Could you check a few things on this model? Use its own coordinates, in mm. Face numbers are marked on the shaded views. A direction names the side the tool comes from. Coordinates: 2 decimals unless noted, no trailing zeros. Loops run counter-clockwise (first coordinate to the right, second up) from the corner with the lowest first, then second, coordinate; pieces in that order, holes last. Notation, with made-up numbers: M 56.5,-16 L 114.5,-16 A8 ccw 114.5,-3 Z; hole C -38.5,23.5 d1. An arc over 180 degrees is marked long. Return JSON: item names as keys, results as strings. Group by question number.
from build123d import *

# Parameters (mm, degrees)
F0_W      = 38.1
F0_H      = 38.1
F1_DEPTH  = 38.1
F6_DEPTH  = 38.1
F8_DEPTH  = 38.1
F9_W      = 25.4
F9_H      = 7.62
F10_DEPTH = 38.1


with BuildPart() as f1:
    # F0 (on Front) → F1 (new body)
    with BuildSketch(Plane.XZ):
        with Locations((19.05, 19.05)):
            Rectangle(F0_W, F0_H)
    extrude(amount=F1_DEPTH)

    # F5 (on offset) → F6 (cut)
    with BuildSketch(Plane.YZ.offset(38.1)):
        Polygon((-11.43, 16.449932), (-6.35, 38.1), (-31.75, 38.1), (-26.67, 16.449932), (-21.59, 28.575), (-16.51, 28.575), align=None)
        Polygon((-6.35, 0), (0, 0), (0, 38.1), align=None)
        Polygon((-19.05, 0), (-12.7, 0), (-19.05, 15.875), (-25.4, 0), align=None)
        Polygon((-31.75, 0), (-38.1, 38.1), (-38.1, 0), align=None)
    extrude(amount=-F6_DEPTH, mode=Mode.SUBTRACT)

    # F7 (on offset) → F8 (cut)
    with BuildSketch(Plane.XZ.offset(38.1)):
        Polygon((11.43, 22.225), (6.35, 0), (31.75, 0), (26.67, 22.225), (21.59, 9.525), (16.51, 9.525), align=None)
        Polygon((25.4, 38.1), (12.7, 38.1), (19.05, 22.225), align=None)
        Polygon((31.75, 38.1), (38.1, 0), (38.1, 38.1), align=None)
        Polygon((0, 38.1), (0, 0), (6.35, 38.1), align=None)
    extrude(amount=-F8_DEPTH, mode=Mode.SUBTRACT)

    # F9 (on offset) → F10 (cut)
    with BuildSketch(Plane.XY.offset(38.1)):
        with Locations((12.7, -26.67)):
            Rectangle(F9_W, F9_H)
        with Locations((25.4, -11.43)):
            Rectangle(F9_W, F9_H)
    extrude(amount=-F10_DEPTH, mode=Mode.SUBTRACT)


solid = f1.part
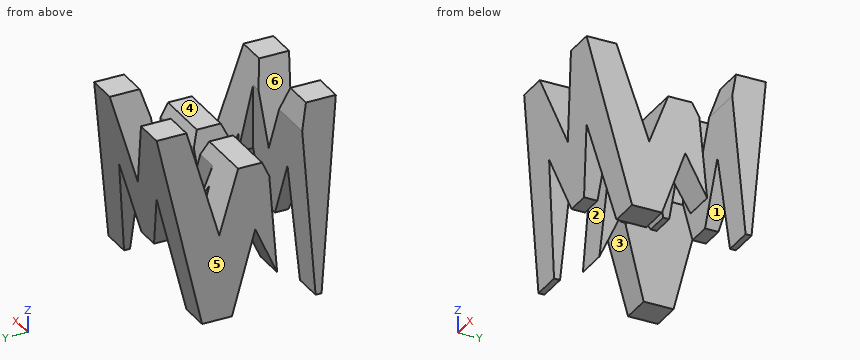
(1) Imagine slicing it at C-C, the plane x = 15.5. Write out the boundary of the cut face in (y, z) (3 decimals).
(2) For the marked faces 1, 2 and 3, which set-ups out of +Z, -Z, +X, -X, +Y, -Y let a thin tool reach every point of the face, with its end or its side?
(3) We'd pull the mould along X, two halves only. Please class the marked faces 4, 5 and 6: +X half, -X half, draft (parallel to the pull), parting line (faces both ways), or undercut.
(4) Will these pins go through, and if not, where does the flat tip stop? P1, Ø5.5, axis at x = 27, y = -18, coming from the +Z side (3 decimals); P2, Ø3.5, axis at y = -29, z = 26, coming from the -X side; P3, Ø1, axis at x = 19.5, y = -15.5, coming from the +Z side.
(5) Imagine slicing it at A-A, the plane z = 35. Write out the boundary of the cut face in (x, y).
(6) If I drill on L1, parallel to Y at x = 5, z = 20; L2, parallel to Y at x = 35, z = 18; L3, parallel to X at y = -32.5, z = 21.5, over which ranges is the centre line in solid material (lowest first)? Write a range as [from, to].
(7) Imagine slicing it at D-D, the plane z = 10.5. Count the separate pieces of the cut face and the enclosed holes in it, then the cut area to 3 significant figures.
Checks:
{
 "1": {"outline": "M -36.933,31.1 L -33.758,12.05 L -30.48,12.05 L -30.48,31.1 Z; M -22.86,12.05 L -20.58,12.05 L -19.05,15.875 L -17.52,12.05 L -15.24,12.05 L -15.24,25.544 L -16.51,28.575 L -21.59,28.575 L -22.86,25.544 Z; M -7.62,12.05 L -4.342,12.05 L -1.167,31.1 L -7.62,31.1 Z"},
 "2": {"face 1": "-Z, +Y, -Y", "face 2": "+Z, -Z, -X", "face 3": "-Z, +X, -X"},
 "3": {"face 4": "draft", "face 5": "-X half", "face 6": "undercut"},
 "4": {"P1": "z = 28.575", "P2": "x = 4.18", "P3": "z = 24.6"},
 "5": {"outline": "M 5.83,-37.58 L 13.94,-37.58 L 13.94,-31.02 L 5.83,-31.02 Z; M 5.83,-7.08 L 13.94,-7.08 L 13.94,-0.52 L 5.83,-0.52 Z; M 24.16,-37.58 L 32.27,-37.58 L 32.27,-31.02 L 24.16,-31.02 Z; M 24.16,-7.08 L 32.27,-7.08 L 32.27,-0.52 L 24.16,-0.52 Z"},
 "6": {"L1": "[-35.08, -30.48], [-22.86, -12.92], [-10.6, -3.02]", "L2": "[-34.75, -27.03], [-26.02, -15.24], [-7.62, -3.35]", "L3": "[3.58, 11.26], [11.72, 26.38], [26.84, 34.52]"},
 "7": {"separate pieces": "10", "enclosed holes": "0", "area": "293 mm²"}
}
